Input: part model. Units: mm. Frame: model coordinates. A direction names the side the tool comes from. Give positions to 0.01 mm unless a question says otherwise; leave off trailing zeros. Write each loop counter-clockwise with the first axis right and the second up, starting at its lowest first coordinate (ties: lowest second). Pieces come first, ordered by that corner, then holes. Notation, with made-up numbers: (69.25, 12.5) - (113.25, 12.5) arc R22 ccw to (113.25, 20.5) - close; hole circle Ø4 at (1, 85). An arc over 180 degrees is marked (long way). Use a Markdown table: item, result. Add a question column.
1. Section query A-A, the plane y = 11.5. Count the separate pieces of the cut face and the enclosed holes in it, plus the area to 3 significant figures.
2. Section query C-C, the plane x = 64. Return loops of the section in (y, z).
3. Pin query (flat end, axial travel): pin 1 (1.9 mm diameter, centred on y = 2, z = 6.5, fed in from +X); pin 2 (2.5 mm diameter, centred on x = -46.5, y = 13, fed in from +Z); pin 3 (6 mm diameter, centred on x = -65.5, y = 5.5, fed in from -Z). Return the tip coordinate at first contact, or that it passes through.
4. Set-up query: faces 1 (the flat face through (-54.07, 3, 6)), 2 (the flat face through (43.889, 34.969, 9.966)). Return all of +Z, -Z, +X, -X, +Y, -Y with unobstructed straight access to the full face (end or side cutting, diameter ignored); none if empty.
5. Mould query, pull axis Y, two halves, no side actions, for faces 3 (the flat face through (-55.07, 3.13, -18)), 4 (the flat face through (32.164, 19, 20)). Classes: released by +Y, released by -Y, zero draft, split by the parting line, or undercut.
6. Material intervals for probe 1 along Y at (x, z) = (-74.5, 2); probe 2 along Z at (x, y) = (-37, 10.5); probe 3 along Z at (x, y) = (26.5, 20), sorted ascending.
7. Section query B-B, the plane x = 23.5. Return loops of the section in (y, z), plus the area to 3 significant figures.
```python
from build123d import *

# Parameters (mm, degrees)
F1_DEPTH  = 19.05
F2_DEPTH  = 19.05
F3_DEPTH  = 12.7
F4_DEPTH  = 6.35
F5_DEPTH  = 6.35
F7_DEPTH  = 6.35
F8_DEPTH  = 6.35
F11_DEPTH = 25.4
F12_DEPTH = 25.4
F6_W      = 1.7239038059
F6_H      = 3.5921024484
F6_W_2    = 1.7933621035
F13_DEPTH = 38.1
F14_DEPTH = 6.35


# Not quite as in the source:
# - a feature names something its author has since deleted; it is built from what else it names


with BuildPart() as f1:
    # F0 (on Front) → F1 (new body)
    with BuildSketch(Plane.XZ):
        Polygon((-75.3014223417, -8.4543359262), (-75.3014223417, -1.435443759), (-78.8935247901, -1.435443759), (-100.7014223417, -1.435443759), (-100.7014223417, -14.135443759), (-75.3014223417, -14.135443759), align=None)
    extrude(amount=-F1_DEPTH)

    # F0 (on Front) → F2 (join)
    with BuildSketch(Plane.XZ):
        Polygon((-68.0739664064, -1.435443759), (-75.3014223417, -1.435443759), (-75.3014223417, -8.4543359262), (-75.3014223417, -14.135443759), (-58.9322418971, -14.135443759), (-55.3401394486, -14.135443759), (-55.3401394486, -1.435443759), (-56.6101394486, -1.435443759), (-62.7698475104, -1.435443759), (-64.1519069584, -1.435443759), (-65.5339664064, -1.435443759), align=None)
        Polygon((-55.3401394486, -1.435443759), (-55.3401394486, -14.135443759), (-36.2901394486, -14.135443759), (-36.2901394486, -1.435443759), (-38.0835015521, -1.435443759), (-54.0701394486, -1.435443759), align=None)
        Polygon((-34.2535879934, -1.435443759), (-36.2901394486, -1.435443759), (-36.2901394486, -14.135443759), (-29.5884479715, -14.0381948012), (-24.5761177188, -13.9654603438), (-18.1276498189, -13.8718859402), (-18.1276498189, -1.435443759), align=None)
    extrude(amount=-F2_DEPTH)



with BuildPart() as f1b:
    # F0 (on Front) → F1, piece 2 (new body)
    with BuildSketch(Plane.XZ):
        Polygon((77.0985776583, -1.435443759), (55.2906801068, -1.435443759), (51.6985776583, -1.435443759), (48.562251594, -1.435443759), (46.022251594, -1.435443759), (44.5195358117, -1.435443759), (43.0168200294, -1.435443759), (33.2472785554, -1.435443759), (31.9772785554, -1.435443759), (31.9772785554, -14.135443759), (35.6239399467, -14.135443759), (77.0985776583, -14.135443759), align=None)
    extrude(amount=-F1_DEPTH)

    # F0 (on Front) → F2, piece 2 (join)
    with BuildSketch(Plane.XZ):
        Polygon((14.2324982387, -13.8718859402), (14.2324982387, -1.435443759), (12.1164883202, -1.435443759), (-5.4276498189, -1.435443759), (-5.4276498189, -13.8718859402), (1.2740385811, -13.8718859402), (7.7840224387, -13.8718859402), align=None)
        Polygon((15.9564020446, -1.435443759), (14.2324982387, -1.435443759), (14.2324982387, -13.8718859402), (31.9772785554, -14.135443759), (31.9772785554, -1.435443759), (30.7072785554, -1.435443759), align=None)
        Polygon((77.0985776583, -1.435443759), (55.2906801068, -1.435443759), (51.6985776583, -1.435443759), (48.562251594, -1.435443759), (46.022251594, -1.435443759), (44.5195358117, -1.435443759), (43.0168200294, -1.435443759), (33.2472785554, -1.435443759), (31.9772785554, -1.435443759), (31.9772785554, -14.135443759), (35.6239399467, -14.135443759), (77.0985776583, -14.135443759), align=None)
    extrude(amount=-F2_DEPTH)


with BuildPart() as f1_1:
    add(f1.part)
    # F3 (add, through all): a face of the model
    f3_faces = [f1b.part.faces().sort_by_distance(p)[0] for p in [
        (-5.4276498189, 9.525, -7.6536648496),
    ]]

    add(f1b.part)  # F3 merges F1b
    extrude(f3_faces, amount=F3_DEPTH)

    # F0 (on Front) → F4 (join)
    with BuildSketch(Plane.XZ):
        Polygon((-78.8935247901, -1.435443759), (-75.3014223417, -1.435443759), (-68.0739664064, 5.7920121763), (-65.5339664064, 8.3320121763), (-58.1879977366, 15.6779808461), (-55.7665104711, 18.0994681116), (-53.9731483676, 18.0994681116), (-37.4634148507, 18.0994681116), (-36.1934148507, 18.0994681116), (-34.9234148507, 18.0994681116), (-13.8379737969, 18.0994681116), (-11.8014223417, 18.0994681116), (-9.6854124232, 18.0994681116), (12.8047038004, 18.0994681116), (14.0747038004, 18.0994681116), (15.3447038004, 18.0994681116), (30.4397619819, 18.0994681116), (32.1636657878, 18.0994681116), (36.2527101199, 14.0104237794), (46.022251594, 4.2408823054), (48.562251594, 1.7008823054), (51.6985776583, -1.435443759), (55.2906801068, -1.435443759), (32.1636657878, 21.69157056), (-55.7665104711, 21.69157056), align=None)
        Polygon((-68.0739664064, 5.7920121763), (-68.0739664064, -1.435443759), (-65.5339664064, -1.435443759), (-65.5339664064, 8.3320121763), align=None)
        Polygon((-36.1934148507, 18.0994681116), (-37.4634148507, 18.0994681116), (-37.4634148507, 1.5401106785), (-36.1934148507, 0.2662933926), align=None)
        Polygon((-34.9234148507, 18.0994681116), (-36.1934148507, 18.0994681116), (-36.1934148507, 0.2662933926), (-34.9234148507, 1.2793859922), align=None)
        Polygon((-11.7776498189, 16.4938528035), (-13.0476498189, 15.4807602039), (-13.0476498189, -1.435443759), (-11.7776498189, -1.435443759), align=None)
        Polygon((-10.5076498189, 15.5408907631), (-11.7776498189, 16.4938528035), (-11.7776498189, -1.435443759), (-10.5076498189, -1.435443759), align=None)
        Polygon((15.3447038004, 18.0994681116), (14.0747038004, 18.0994681116), (14.0747038004, 0.2707367444), (15.3447038004, 1.6543241772), align=None)
        Polygon((14.0747038004, 18.0994681116), (12.8047038004, 18.0994681116), (12.8047038004, 1.2236987848), (14.0747038004, 0.2707367444), align=None)
        Polygon((30.7072785554, -1.435443759), (31.9772785554, -1.435443759), (31.9772785554, 16.0183226994), (30.7072785554, 14.6347352666), align=None)
        Polygon((31.9772785554, 16.0183226994), (31.9772785554, -1.435443759), (33.2472785554, -1.435443759), (33.2472785554, 14.0104237794), align=None)
        Polygon((-55.3401394486, 15.8730630517), (-55.3401394486, -1.435443759), (-54.0701394486, -1.435443759), (-54.0701394486, 14.5992457658), align=None)
        Polygon((-56.6101394486, 12.9144267948), (-56.6101394486, -1.435443759), (-55.3401394486, -1.435443759), (-55.3401394486, 15.8730630517), align=None)
    extrude(amount=-F4_DEPTH)

    # F0 (on Front) → F5 (join)
    with BuildSketch(Plane.XZ):
        Polygon((-55.7665104711, 18.0994681116), (-64.1519069584, -1.435443759), (-62.7698475104, -1.435443759), (-56.6101394486, 12.9144267948), (-55.3401394486, 15.8730630517), (-54.0701394486, 14.5992457658), (-38.0835015521, -1.435443759), (-36.2901394486, -1.435443759), align=None)
        Polygon((-58.1879977366, 15.6779808461), (-65.5339664064, -1.435443759), (-64.1519069584, -1.435443759), (-55.7665104711, 18.0994681116), align=None)
        Polygon((-53.9731483676, 18.0994681116), (-55.7665104711, 18.0994681116), (-36.2901394486, -1.435443759), (-11.8014223417, 18.0994681116), (-13.8379737969, 18.0994681116), (-34.9234148507, 1.2793859922), (-36.1934148507, 0.2662933926), (-37.4634148507, 1.5401106785), align=None)
        Polygon((-11.8014223417, 18.0994681116), (-36.2901394486, -1.435443759), (-34.2535879934, -1.435443759), (-13.0476498189, 15.4807602039), (-11.7776498189, 16.4938528035), (-10.5076498189, 15.5408907631), (12.1164883202, -1.435443759), (14.2324982387, -1.435443759), align=None)
        Polygon((-9.6854124232, 18.0994681116), (-11.8014223417, 18.0994681116), (14.2324982387, -1.435443759), (32.1636657878, 18.0994681116), (30.4397619819, 18.0994681116), (15.3447038004, 1.6543241772), (14.0747038004, 0.2707367444), (12.8047038004, 1.2236987848), align=None)
    extrude(amount=-F5_DEPTH)

    # F0 (on Front) → F7 (join)
    with BuildSketch(Plane.XZ):
        Polygon((-55.3401394486, -14.135443759), (-58.9322418971, -14.135443759), (-51.0965817995, -21.9711038566), (28.7455422806, -20.8125063022), (35.6239399467, -14.135443759), (31.9772785554, -14.135443759), (28.8399389893, -17.1809513785), (27.7001179184, -18.2874091537), (20.2112810939, -18.3960804614), (-6.4368105921, -18.782773754), (-11.1798369081, -18.8516003134), (-15.855044379, -18.9194427462), (-43.0566496336, -19.3141681332), (-50.0597917346, -19.415791473), (-51.1394793261, -18.3361038815), align=None)
        Polygon((-26.606417659, -14.7384993405), (-50.0597917346, -19.415791473), (-43.0566496336, -19.3141681332), (-26.647951981, -16.0417915366), (-15.855044379, -18.9194427462), (-11.1798369081, -18.8516003134), align=None)
        Polygon((-29.5884479715, -14.0381948012), (-51.1394793261, -18.3361038815), (-50.0597917346, -19.415791473), (-26.606417659, -14.7384993405), (-11.1798369081, -18.8516003134), (3.6282092287, -14.5043621946), (27.7001179184, -18.2874091537), (28.8399389893, -17.1809513785), (7.7840224387, -13.8718859402), (1.2740385811, -13.8718859402), (-11.1963136804, -17.5328409511), (-24.5761177188, -13.9654603438), align=None)
        Polygon((3.6282092287, -14.5043621946), (-11.1798369081, -18.8516003134), (-6.4368105921, -18.782773754), (3.7125368777, -15.8032023917), (20.2112810939, -18.3960804614), (27.7001179184, -18.2874091537), align=None)
    extrude(amount=-F7_DEPTH)

    # F0 (on Front) → F8 (join)
    with BuildSketch(Plane.XZ):
        Polygon((46.022251594, -1.435443759), (48.562251594, -1.435443759), (48.562251594, 1.7008823054), (46.022251594, 4.2408823054), align=None)
    extrude(amount=-F8_DEPTH)

    # F9: F1 across face


with BuildPart() as f1_2:
    add(f1_1.part)
    add(f1_1.part.mirror(Plane(origin=(-11.8589412224, 19.05, -7.7486185811), x_dir=(-1, 0, 0), z_dir=(0, 1, 0))))

    # F10 (on face) → F11 (join, through all)
    with BuildSketch(Plane.XZ.offset(-31.75)):
        Polygon((20.248135424, -20.9358130769), (28.7455422806, -20.8125063022), (28.7086879505, -18.2727736867), (20.2112810939, -18.3960804614), align=None)
    extrude(amount=F11_DEPTH)

    # F10 (on face) → F12 (join, through all)
    with BuildSketch(Plane.XZ.offset(-31.75)):
        Polygon((-43.0566496336, -21.8544355458), (-43.0566496336, -19.3141681332), (-51.0965817995, -19.3141681332), (-51.0965817995, -19.325645402), (-51.0965817995, -21.9711038566), align=None)
    extrude(amount=F12_DEPTH)

    # F6 (on face) → F13 (join)
    with BuildSketch(Plane.XZ):
        Polygon((15.3447038004, 18.0994681116), (15.3447038004, 21.69157056), (12.8047038004, 21.69157056), (12.8047038004, 18.0994681116), (14.0747038004, 18.0994681116), align=None)
        with Locations((31.3017138849, 19.8955193358)):
            Rectangle(F6_W, F6_H)
        with Locations((-54.8698294194, 19.8955193358)):
            Rectangle(F6_W_2, F6_H)
        Polygon((-34.9234148507, 18.0994681116), (-34.9234148507, 21.69157056), (-37.4634148507, 21.69157056), (-37.4634148507, 18.0994681116), (-36.1934148507, 18.0994681116), align=None)
    extrude(amount=-F13_DEPTH)

    # F0 (on Front) → F14 (join)
    with BuildSketch(Plane.XZ):
        Polygon((32.1636657878, 18.0994681116), (14.2324982387, -1.435443759), (15.9564020446, -1.435443759), (30.7072785554, 14.6347352666), (31.9772785554, 16.0183226994), (33.2472785554, 14.0104237794), (43.0168200294, -1.435443759), (44.5195358117, -1.435443759), align=None)
        Polygon((44.5195358117, -1.435443759), (46.022251594, -1.435443759), (36.2527101199, 14.0104237794), (32.1636657878, 18.0994681116), align=None)
    extrude(amount=-F14_DEPTH)


solid = f1_2.part
```
Result sheet:
| question | item | result |
|---|---|---|
| 1 | separate pieces | 7 |
| 1 | enclosed holes | 0 |
| 1 | area | 2,320 mm² |
| 2 | outline | (0, -14.14) - (38.1, -14.14) - (38.1, -1.44) - (0, -1.44) - close |
| 3 | pin 1 | stops at x = 48.31 |
| 3 | pin 2 | stops at z = -1.44 |
| 3 | pin 3 | stops at z = -14.14 |
| 4 | face 1 | +Y, -Y |
| 4 | face 2 | +Z, +X, +Y, -Y |
| 5 | face 3 | zero draft |
| 5 | face 4 | undercut |
| 6 | probe 1 | y = 0 to 6.35, 31.75 to 38.1 |
| 6 | probe 2 | z = -14.14 to -1.44, 18.1 to 21.69 |
| 6 | probe 3 | z = -20.85 to -18.3, -14.05 to -1.44 |
| 7 | outline | (0, -20.89) - (38.1, -20.89) - (38.1, -16.34) - (31.75, -16.34) - (31.75, -18.35) - (6.35, -18.35) - (6.35, -16.34) - (0, -16.34) - close; (0, -14.01) - (38.1, -14.01) - (38.1, -1.44) - (0, -1.44) - close; (0, 6.78) - (6.35, 6.78) - (6.35, 10.54) - (0, 10.54) - close; (0, 18.1) - (6.35, 18.1) - (6.35, 21.69) - (0, 21.69) - close; (31.75, 8.66) - (38.1, 8.66) - (38.1, 10.54) - (31.75, 10.54) - close; (31.75, 18.1) - (38.1, 18.1) - (38.1, 21.69) - (31.75, 21.69) - close |
| 7 | area | 683 mm² |
